```python
from build123d import *

# Parameters (mm, degrees)
SKETCH6_R                = 1.65
BOSS_EXTRUDE3_DEPTH      = 14.75
SKETCH9_W                = 26.5
SKETCH9_H                = 6
BOSS_EXTRUDE4_DEPTH      = 103.75
BOSS_EXTRUDE6_DEPTH      = 6.75
BOSS_EXTRUDE6_DEPTH_BACK = 33.25
SKETCH14_W               = 12
SKETCH14_H               = 6
SKETCH10_R               = 1.7
CUT_EXTRUDE1_DEPTH       = 107.021813793
SKETCH11_W               = 23.3
SKETCH11_H               = 23.3
CUT_EXTRUDE2_DEPTH       = 4
SKETCH12_W               = 36.472759933
SKETCH12_H               = 9.4
CUT_EXTRUDE3_DEPTH       = 4
SKETCH15_W               = 91.75
SKETCH15_H               = 6
BOSS_EXTRUDE8_DEPTH      = 30


with BuildPart() as part:
    # Sketch6 → Boss-Extrude3 (new body)
    with BuildSketch(Plane(origin=(0, 0, 0), x_dir=(1, 0, 0), z_dir=(0, 1, 0))):
        Polygon((-13.25, 3.3), (-13.25, 0), (13.25, 0), (13.25, 3.3), (13.25, 33), (-13.25, 33), align=None)
        with Locations(Location((8, 10.85, 0), (0, 0, 270))):
            Circle(SKETCH6_R, mode=Mode.SUBTRACT)
        with Locations(Location((8, 24.85, 0), (0, 0, 270))):
            Circle(SKETCH6_R, mode=Mode.SUBTRACT)
        with Locations(Location((-8, 24.85, 0), (0, 0, 270))):
            Circle(SKETCH6_R, mode=Mode.SUBTRACT)
        with Locations(Location((-8, 10.85, 0), (0, 0, 270))):
            Circle(SKETCH6_R, mode=Mode.SUBTRACT)
    extrude(amount=BOSS_EXTRUDE3_DEPTH)

    # Sketch9 → Boss-Extrude4 (add)
    with BuildSketch(Plane.XY):
        with Locations((0, 3)):
            Rectangle(SKETCH9_W, SKETCH9_H)
    extrude(amount=BOSS_EXTRUDE4_DEPTH)

    # Sketch14 → Boss-Extrude6 (add, two sides: drawn at the far end of the back side and taken through both)
    with BuildSketch(Plane.ZY.offset(13.25).offset(-BOSS_EXTRUDE6_DEPTH_BACK)):
        with Locations((97.75, 3)):
            Rectangle(SKETCH14_W, SKETCH14_H)
    extrude(amount=BOSS_EXTRUDE6_DEPTH + BOSS_EXTRUDE6_DEPTH_BACK)

    # Sketch10 → Cut-Extrude1 (cut, through all)
    with BuildSketch(Plane(origin=(0, 6, 0), x_dir=(1, 0, 0), z_dir=(0, 1, 0))):
        with Locations(Location((-15, -97.75, 0), (0, 0, 270))):
            Circle(SKETCH10_R)
        with Locations(Location((15, -97.75, 0), (0, 0, 270))):
            Circle(SKETCH10_R)
    extrude(amount=-CUT_EXTRUDE1_DEPTH, mode=Mode.SUBTRACT)

    # Sketch11 → Cut-Extrude2 (cut)
    with BuildSketch(Plane.XZ):
        with Locations((0, -17.85)):
            Rectangle(SKETCH11_W, SKETCH11_H)
    extrude(amount=-CUT_EXTRUDE2_DEPTH, mode=Mode.SUBTRACT)

    # Sketch12 → Cut-Extrude3 (cut)
    with BuildSketch(Plane.XZ):
        with Locations((-0.463620034, 97.75)):
            Rectangle(SKETCH12_W, SKETCH12_H)
    extrude(amount=-CUT_EXTRUDE3_DEPTH, mode=Mode.SUBTRACT)

    # Sketch15 → Boss-Extrude8 (add)
    with BuildSketch(Plane(origin=(13.25, 0, 0), x_dir=(0, 0, -1), z_dir=(1, 0, 0))):
        with Locations((-45.875, 3)):
            Rectangle(SKETCH15_W, SKETCH15_H)
    extrude(amount=BOSS_EXTRUDE8_DEPTH)


solid = part.part
```
Geometry check sheet. Reference: the model listing, model coordinates, mm. A direction names the side the tool comes from. Give positions to 0.01 mm unless a question says otherwise; leave off trailing zeros. Order: outer loops, then holes, each group sorted by start corner. A loop starts at its lowest first (then second) coordinate and runs counter-clockwise, first axis right, second up.
1. Section check B-B, the plane y = 10.5. Enter the section's corners in (x, z).
2. Section check A-A, the plane x = -8. Enter the section's corners in (y, z).
3. Section check D-D, the plane x = 15. Enter the section's corners in (y, z).
4. Section check C-C, the plane z = 97.75. Enter the section's corners in (x, y), and give its area (3 significant figures).
5. Access from +Z, -Z, +X, -X, +Y, -Y to the whole of each face (thin tool, end or side, straight path). Record for faces 1 (the face through (11, 6, 53)), 2 (the face through (28, 3, 0)), 3 (the face through (0, 4, -18)).
6. Thickness scan on L1, parallel to X at y = 12, z = -10.85; L2, parallel to X at y = 13, z = -24; L3, parallel to X at y = 5.5, z = 76.5. Record the ranges inside material, lowest first.
7. Release check for a two-part mould opening along Z. For faces 4 (the face through (43.25, 3, 47)), 5 (the face through (-1, 4, 98)), 6 (the face through (0, 3, 103.75)) record: pulls with the +Z half, pulls with the -Z half, needs draft (parallel to the pull), parting line crosses it, or undercut.
8. Gauge pin test, flat ends, axial feed: pin 1 Ø3 at (x, y) = (33.5, 1.5) entering from -Z; pin 2 Ø2 at (y, z) = (2, 98) entering from +X; pin 3 Ø2 at (x, z) = (-15, 97.75) entering from -Y; pin 4 Ø3 at (x, z) = (2.5, 99.5) entering from -Y. Record the tip position at first contact, or that the pin passes through.
Values follow:
1. outline: (-13.25, -33) - (13.25, -33) - (13.25, 0) - (-13.25, 0) - close; hole circle Ø3.3 at (-8, -24.85); hole circle Ø3.3 at (-8, -10.85); hole circle Ø3.3 at (8, -24.85); hole circle Ø3.3 at (8, -10.85)
2. outline: (0, -33) - (14.75, -33) - (14.75, -26.5) - (4, -26.5) - (4, -29.5) - (0, -29.5) - close; (0, -6.2) - (4, -6.2) - (4, -9.2) - (14.75, -9.2) - (14.75, 0) - (6, 0) - (6, 103.75) - (0, 103.75) - (0, 102.45) - (4, 102.45) - (4, 93.05) - (0, 93.05) - close; (4, -23.2) - (14.75, -23.2) - (14.75, -12.5) - (4, -12.5) - close
3. outline: (0, 0) - (6, 0) - (6, 96.05) - (4, 96.05) - (4, 93.05) - (0, 93.05) - close; (0, 102.45) - (4, 102.45) - (4, 99.45) - (6, 99.45) - (6, 103.75) - (0, 103.75) - close
4. outline: (-20, 0) - (-18.7, 0) - (-18.7, 4) - (-16.7, 4) - (-16.7, 6) - (-20, 6) - close; (-13.3, 4) - (13.3, 4) - (13.3, 6) - (-13.3, 6) - close; (16.7, 4) - (17.77, 4) - (17.77, 0) - (20, 0) - (20, 6) - (16.7, 6) - close
4. area: 80.5 mm2
5. face 1: +Z, +X, -X, +Y
5. face 2: -Z, +X, +Y, -Y
5. face 3: -Y
6. L1: x = -13.25 to -9.65, -6.35 to 6.35, 9.65 to 13.25
6. L2: x = -13.25 to -9.41, -6.59 to 6.59, 9.41 to 13.25
6. L3: x = -13.25 to 43.25
7. face 4: needs draft
7. face 5: undercut
7. face 6: pulls with the +Z half
8. pin 1: stops at z = 0
8. pin 2: stops at x = 20
8. pin 3: passes through
8. pin 4: stops at y = 4
